Build history of the part. All positions in model axes, mm. Face numbers are marked on the shaded views. A direction names the side the tool comes from. Round coordinates to 2 decimals unless told otherwise and drop trailing zeros. Loops run counter-clockwise (first coordinate to the right, second up) from the corner with the lowest first, then second, coordinate; pieces in that order, holes last. Notation, with made-up numbers: M 49,24.5 L 93,24.5 A19 cw 93,47.5 Z; hole C 75,42.5 d9. An arc over 180 degrees is marked long. Write each question's results on one line, items separated by ' | '. Start each with the question number.
```python
from build123d import *

# Parameters (mm, degrees)
SKETCH020_R     = 86
POCKET013_DEPTH = 25
CHAMFER003_SIZE = 0.5


with BuildPart() as part:
    # Sketch019 → Revolution (revolve)
    with BuildSketch(Plane.XZ):
        Polygon((85, 0), (85, 28.5), (84.5, 29), (87, 29), (87, 0), align=None)
    revolve(axis=Axis((0, 0, 0), (0, 0, 1)))

    # Sketch020 (on Face5 of Revolution) → Pocket013 (cut)
    with BuildSketch(Plane(origin=(0, 0, 0), x_dir=(1, 0, 0), z_dir=(0, 0, -1))):
        Circle(SKETCH020_R)
    extrude(amount=-POCKET013_DEPTH, mode=Mode.SUBTRACT)

    # Chamfer003
    chamfer003_edges = [part.edges().sort_by_distance(p)[0] for p in [
        (-85, 0, 25),
        (-86, 0, 0),
    ]]
    chamfer(chamfer003_edges, length=CHAMFER003_SIZE)


solid = part.part
```
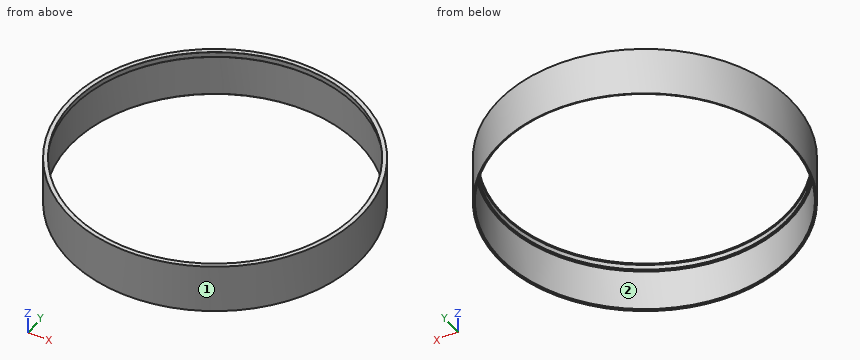
Item 1: Saw through at A-A, the plane y = 0. Give the cut face in (x, z).
Item 2: Tool access for the marked faces 1 and 2: list every direction of +Z, -Z, +X, -X, +Y, -Y with a clear straight run to the whole face (end or side of a thin tool).
Item 3: Drill centre lines: line 1 along Y through (x, z) = (0, 27.4); line 2 along Y through (x, z) = (0, 8.5); line 3 along X through (y, z) = (44, 26.5). Where is each one in solid material? Low to high. Write a range as [from, to].
Item 4: Saw through at C-C, the plane z = 20.75. Give the cut face in (x, y), then the cut area to 3 significant figures.
Item 5: Drop flat-ended pins along their axis: pin 1 (10 mm diameter, centred on x = 37.5, z = 16.5, fed in from -Y); pin 2 (1 mm diameter, centred on x = 13, z = 12, fed in from +Y); pin 3 (8 mm diameter, centred on y = 46, z = 11, fed in from -X); pin 4 (10 mm diameter, centred on x = -41.5, y = -62, fed in from -Z). Give the stop position or say it passes through.
Working result:
1) outline: M -87,0 L -86.5,0 L -86,0.5 L -86,25 L -85.5,25 L -85,25.5 L -85,28.5 L -84.5,29 L -87,29 Z; M 84.5,29 L 85,28.5 L 85,25.5 L 85.5,25 L 86,25 L 86,0.5 L 86.5,0 L 87,0 L 87,29 Z
2) face 1: +Z, -Z | face 2: -Z
3) line 1: y = [-87, -85], [85, 87] | line 2: y = [-87, -86], [86, 87] | line 3: x = [-75.05, -72.73], [72.73, 75.05]
4) outline: C 0,0 d174; hole C 0,0 d172 | area: 543 mm²
5) pin 1: stops at y = -80.7 | pin 2: stops at y = 86.1 | pin 3: stops at x = -76.19 | pin 4: passes through
